from build123d import *

# Parameters (mm, degrees)
BOSS_EXTRUDE1_DEPTH = 1
BOSS_EXTRUDE2_START = 7
BOSS_EXTRUDE2_DEPTH = 7
SKETCH2_W           = 2.5
SKETCH2_H           = 4.000000000000001
CUT_EXTRUDE1_DEPTH  = 1
CUT_EXTRUDE2_DEPTH  = 4.5
BOSS_EXTRUDE3_START = 7
BOSS_EXTRUDE3_DEPTH = 7
SKETCH4_R           = 1.2500000000000002
CUT_EXTRUDE3_DEPTH  = 11
CIRPATTERN1_COUNT   = 3


with BuildPart() as part:
    # Sketch1 → Boss-Extrude1 (new body)
    with BuildSketch(Plane(origin=(0, 0, 0), x_dir=(1, 0, 0), z_dir=(0, 1, 0))):
        with BuildLine():
            ThreePointArc((-10.500000000000004, 41.502362583351804), (-42.81, 5.24e-15), (-10.499999999999995, -41.50236258335181))
            Line((-10.5, -41.5023625833518), (-10.5, 41.50236258335181))
        make_face()
        with BuildLine():
            Line((-10.5, 41.50236258335181), (-10.5, -41.5023625833518))
            ThreePointArc((-10.499999999999995, -41.50236258335181), (-7.86e-15, -42.81), (10.499999999999979, -41.50236258335181))
            Line((10.500000000000002, -41.5023625833518), (10.500000000000002, 41.50236258335181))
            ThreePointArc((10.499999999999998, 41.502362583351804), (2.62e-15, 42.81), (-10.500000000000004, 41.502362583351804))
        make_face()
        with BuildLine():
            Line((10.500000000000002, 41.50236258335181), (10.500000000000002, -41.5023625833518))
            ThreePointArc((10.499999999999979, -41.50236258335181), (33.78017983966337, -26.298204311321346), (42.81, -1.049e-14))
            ThreePointArc((42.81, 0), (33.780179839663376, 26.29820431132134), (10.499999999999998, 41.502362583351804))
        make_face()
    extrude(amount=-BOSS_EXTRUDE1_DEPTH)

    # Sketch1_3 → Boss-Extrude2 (add)
    with BuildSketch(Plane(origin=(0, 0, 0), x_dir=(1, 0, 0), z_dir=(0, 1, 0)).offset(BOSS_EXTRUDE2_START)):
        with BuildLine():
            Line((10.500000000000002, 41.50236258335181), (10.500000000000002, -41.5023625833518))
            ThreePointArc((10.499999999999979, -41.50236258335181), (33.78017983966337, -26.298204311321346), (42.81, -1.049e-14))
            ThreePointArc((42.81, 0), (33.780179839663376, 26.29820431132134), (10.499999999999998, 41.502362583351804))
        make_face()
        with BuildLine():
            ThreePointArc((-10.500000000000004, 41.502362583351804), (-42.81, 5.24e-15), (-10.499999999999995, -41.50236258335181))
            Line((-10.5, -41.5023625833518), (-10.5, 41.50236258335181))
        make_face()
    extrude(amount=-BOSS_EXTRUDE2_DEPTH)

    # Sketch2 → Cut-Extrude1 (cut)
    with BuildSketch(Plane(origin=(0, 7, 0), x_dir=(1, 0, 0), z_dir=(0, 1, 0))):
        with BuildLine():
            Line((-37.85326868955399, -5.000000000000004), (-42.51700953736046, -5.000000000000006))
            ThreePointArc((-42.517009537360465, -5.000000000000005), (-42.23252256285123, -7.0078625827181975), (-41.853268689553985, -9))
            Line((-41.85326868955399, -9.000000000000004), (-37.85326868955399, -9.000000000000004))
            Line((-37.85326868955399, -9.000000000000007), (-37.85326868955399, -5.000000000000004))
        make_face()
        with BuildLine():
            Line((-37.85326868955399, 8.999999999999996), (-41.85326868955399, 8.999999999999996))
            ThreePointArc((-41.853268689554, 8.999999999999995), (-42.232522562851244, 7.007862582718188), (-42.517009537360465, 4.9999999999999964))
            Line((-42.51700953736046, 4.999999999999996), (-37.85326868955399, 4.999999999999996))
            Line((-37.85326868955399, 4.999999999999996), (-37.85326868955399, 8.999999999999996))
        make_face()
        with Locations((-21.10326868955399, 6.9999999999999964)):
            Rectangle(SKETCH2_W, SKETCH2_H)
        Polygon((-19.853268689553985, -9.000000000000004), (-19.853268689553985, -5), (-22.35326868955399, -5.000000000000001), (-22.353268689553985, -9.000000000000004), align=None)
    extrude(amount=-CUT_EXTRUDE1_DEPTH, mode=Mode.SUBTRACT)

    # Sketch2_3 → Cut-Extrude2 (cut)
    with BuildSketch(Plane(origin=(0, 7, 0), x_dir=(1, 0, 0), z_dir=(0, 1, 0))):
        with BuildLine():
            Line((-22.35326868955399, 8.999999999999996), (-37.85326868955399, 8.999999999999996))
            Line((-37.85326868955399, 8.999999999999996), (-37.85326868955399, 4.999999999999996))
            Line((-37.85326868955399, 4.999999999999996), (-42.51700953736046, 4.999999999999996))
            ThreePointArc((-42.517009537360465, 4.9999999999999964), (-42.81, -3.55e-15), (-42.517009537360465, -5.000000000000005))
            Line((-42.51700953736046, -5.000000000000006), (-37.85326868955399, -5.000000000000004))
            Line((-37.85326868955399, -5.000000000000004), (-37.85326868955399, -9.000000000000007))
            Line((-37.85326868955399, -9.000000000000004), (-22.353268689553985, -9.000000000000004))
            Line((-22.353268689553985, -9.000000000000004), (-22.35326868955399, -5.000000000000001))
            Line((-22.35326868955399, -5.000000000000001), (-19.85326868955399, -5.000000000000001))
            Line((-19.853268689553985, -5), (-19.85326868955399, 4.999999999999996))
            Line((-19.85326868955399, 4.999999999999996), (-22.35326868955399, 4.999999999999996))
            Line((-22.35326868955399, 4.999999999999996), (-22.35326868955399, 8.999999999999996))
        make_face()
    extrude(amount=-CUT_EXTRUDE2_DEPTH, mode=Mode.SUBTRACT)

    # Sketch3 → Boss-Extrude3 (add)
    with BuildSketch(Plane(origin=(0, 0, 0), x_dir=(1, 0, 0), z_dir=(0, 1, 0)).offset(BOSS_EXTRUDE3_START)):
        with BuildLine():
            Line((-10.500000000000002, 41.502362583351804), (-10.500000000000002, 39))
            Line((-10.5, 39), (10.5, 39))
            Line((10.499999999999998, 39.00000000000001), (10.499999999999998, 41.502362583351804))
            ThreePointArc((10.499999999999998, 41.502362583351804), (0, 42.809999999999995), (-10.500000000000002, 41.502362583351804))
        make_face()
        with BuildLine():
            Line((10.5, -39), (-10.5, -39))
            Line((-10.5, -39.00000000000001), (-10.5, -41.50236258335179))
            ThreePointArc((-10.500000000000004, -41.50236258335181), (-1.288e-14, -42.81), (10.499999999999982, -41.502362583351825))
            Line((10.499999999999979, -41.502362583351804), (10.499999999999979, -39))
        make_face()
    extrude(amount=-BOSS_EXTRUDE3_DEPTH)

    # Sketch4 → Cut-Extrude3 (cut)
    with BuildSketch(Plane(origin=(42.81, 0, 0), x_dir=(0, 0, -1), z_dir=(1, 0, 0))):
        with Locations((0, 4)):
            Circle(SKETCH4_R)
    cut_extrude3 = extrude(amount=-CUT_EXTRUDE3_DEPTH, mode=Mode.SUBTRACT)

    # CirPattern1: Cut-Extrude3 ×3 about axis
    cirpattern1_axis = Axis((-4.63e-15, 0, -8.01e-15), (0, 1, 0))
    for i in range(1, CIRPATTERN1_COUNT):
        add(cut_extrude3.rotate(cirpattern1_axis, i * 360 / CIRPATTERN1_COUNT), mode=Mode.SUBTRACT)


solid = part.part
Read the model definition and answer for the solid it produces. Units are mm, in the model's axes. A direction names the side the tool comes from. Coordinates: 2 decimals unless noted, no trailing zeros. Order: outer loops, then holes, each group sorted by start corner. A loop starts at its lowest first (then second) coordinate and runs counter-clockwise, first axis right, second up. Notation, with made-up numbers: M -30.5,52 L 18.5,52 A34 ccw 18.5,87 Z; hole C 7.5,-32 d2. An arc over 180 degrees is marked long. Put each result on its own line as item: value. Start each with the question number.
Item 1: Section B-B, the plane y = 4 is taken. Determine the outline of the cut face in (x, z).
Item 2: Given pin 1 Ø3 at (x, y) = (-39.5, 3.5) entering from +Z; pin 2 Ø4 at (y, z) = (4, -8) entering from -X; pin 3 Ø1.8 at (y, z) = (4, 7) entering from +X; pin 4 Ø4 at (x, z) = (-30.5, -32.5) entering from -Y, each flat-ended and moving along its own axis, determine where each tip first touches the part or whether it passes through.
Item 3: Section D-D, the plane z = -20.5 is taken. Determine the outline of the cut face in (x, y).
Item 4: Section A-A, the plane z = 0 is taken. Determine the outline of the cut face in (x, y), plus the area to 3 significant figures.
Item 5: Section C-C, the plane x = 0 is taken. Determine the outline of the cut face in (y, z), plus the area to 3 significant figures.
Item 6: The mould has two halves that part along Y. Classify faces 1 (the face through (-31, 5, 9)), 2 (the face through (-40, 6, -7)), 3 (the face through (-15.92, 4.02, 27.54)): +Y half, -Y half, draft (parallel to the pull), parting line (faces both ways), or undercut.
Item 7: For faces 4 (the face through (-18.46, 2.78, -32.51)), 5 (the face through (19, 7, -1)), 6 (the face through (-22.353, 4, -7)), 7 (the face through (-21, 4, -5)), 8 (the face through (37.39, 2.78, 0.27)), determine the directions among +Z, -Z, +X, -X, +Y, -Y from which every point of the face is accessible in a straight line to the end or side of a thin tool.
Item 8: Consider probe 1 along Y at (x, z) = (37, 0); probe 2 along X at (y, z) = (5, 6); probe 3 along Z at (x, y) = (1, 5.25). Determine where each line is inside the solid, lowest interval first. Write a range as [from, to].
Computed:
1. outline: M -42.52,-5 A42.81 ccw -22.48,-36.43 L -16.99,-26.92 L -14.82,-28.17 L -20.31,-37.68 A42.81 ccw 42.79,-1.25 L 31.81,-1.25 L 31.81,1.25 L 42.79,1.25 A42.81 ccw -20.31,37.68 L -14.82,28.17 L -16.99,26.92 L -22.48,36.43 A42.81 ccw -42.52,5 L -37.85,5 L -37.85,9 L -22.35,9 L -22.35,5 L -19.85,5 L -19.85,-5 L -22.35,-5 L -22.35,-9 L -37.85,-9 L -37.85,-5 Z; hole M -10.5,-39 L 10.5,-39 L 10.5,39 L -10.5,39 Z
2. pin 1: stops at z = 19.72
2. pin 2: stops at x = -42.39
2. pin 3: stops at x = 42.37
2. pin 4: stops at y = -1
3. outline: M -37.58,-1 L 37.58,-1 L 37.58,7 L 10.5,7 L 10.5,0 L -10.5,0 L -10.5,7 L -37.58,7 Z
4. outline: M -42.81,-1 L 42.81,-1 L 42.81,2.75 L 31.81,2.75 L 31.81,5.25 L 42.81,5.25 L 42.81,7 L 10.5,7 L 10.5,0 L -10.5,0 L -10.5,7 L -19.85,7 L -19.85,2.5 L -42.81,2.5 Z
4. area: 407 mm2
5. outline: M -1,-42.81 L 7,-42.81 L 7,-39 L 0,-39 L 0,39 L 7,39 L 7,42.81 L -1,42.81 Z
5. area: 139 mm2
6. face 1: draft
6. face 2: +Y half
6. face 3: undercut
7. face 4: none
7. face 5: +Z, -Z, +X, -X, +Y
7. face 6: +Y
7. face 7: -X, +Y
7. face 8: +X
8. probe 1: y = [-1, 2.75], [5.25, 7]
8. probe 2: x = [-42.39, -37.85], [-22.35, -10.5], [10.5, 42.39]
8. probe 3: z = [-42.8, -39], [39, 42.8]
